from build123d import *

# Parameters (mm, degrees)
F0_R      = 6.35
F1_DEPTH  = 19.05
F3_D      = 5.08
F8_D      = 3.175
F8_DEPTH  = 2.54
F8_TIP    = 0.9538662327
F9_D      = 3.175
F9_DEPTH  = 2.54
F9_TIP    = 0.9538662327
F11_D     = 11.938
F11_DEPTH = 12.7
F11_TIP   = 3.586537035


# Not quite as in the source:
# - the program builds the solid bodies; features that only make, move or delete a surface that nothing else refers to are left out


with BuildPart() as f1:
    # F0 (on Top) → F1 (new body)
    with BuildSketch(Plane.XY):
        Circle(F0_R)
    extrude(amount=F1_DEPTH)

    # F3 (through all)
    with Locations(Plane(origin=(0, 0, 0), x_dir=(1, 0, 0), z_dir=(0, 0, -1))):
        with Locations((0, 0)):
            Hole(F3_D / 2)

    # F8
    with Locations(Plane.XY.offset(19.05)):
        with Locations((0, 4.4337138534)):
            Hole(F8_D / 2, depth=F8_DEPTH)
            with Locations((0, 0, -(F8_DEPTH + F8_TIP / 2))):  # 118° drill point
                Cone(0, F8_D / 2, F8_TIP, mode=Mode.SUBTRACT)

    # F9
    with Locations(Plane.XY.offset(19.05)):
        with Locations((0, -4.445)):
            Hole(F9_D / 2, depth=F9_DEPTH)
            with Locations((0, 0, -(F9_DEPTH + F9_TIP / 2))):  # 118° drill point
                Cone(0, F9_D / 2, F9_TIP, mode=Mode.SUBTRACT)

    # F11
    with Locations(Plane(origin=(0, 0, 0), x_dir=(1, 0, 0), z_dir=(0, 0, -1))):
        with Locations((0, 0)):
            Hole(F11_D / 2, depth=F11_DEPTH)
            with Locations((0, 0, -(F11_DEPTH + F11_TIP / 2))):  # 118° drill point
                Cone(0, F11_D / 2, F11_TIP, mode=Mode.SUBTRACT)


solid = f1.part
The listing builds one solid part. Answer for the finished solid, in the listing's coordinates (mm). A direction names the side the tool comes from. Give positions to 0.01 mm unless a question says otherwise; leave off trailing zeros. Write each loop counter-clockwise with the first axis right and the second up, starting at its lowest first coordinate (ties: lowest second). Pieces come first, ordered by that corner, then holes. Notation, with made-up numbers: (81.25, -30) -> (112.25, -30) arc R28 cw to (112.25, 1) -> close; hole circle Ø10 at (51.5, 43.25). An arc over 180 degrees is marked (long way). Use a Markdown table: item, result.
(1) Find the intervals of material crossed by probe 1 along Y at (x, z) = (0, 17.9); probe 2 along Y at (x, z) = (0, 3.5); probe 3 along Y at (x, z) = (0, 15.9), in increasing order. Write a range as from..to.
Return value:
| item | result |
|---|---|
| probe 1 | -6.35..-6.03, -2.86..-2.54, 2.54..2.85, 6.02..6.35 |
| probe 2 | -6.35..-5.97, 5.97..6.35 |
| probe 3 | -6.35..-5.02, -3.87..-2.54, 2.54..3.86, 5.01..6.35 |
(2) Section A-A, the plane y = 0 is taken. Determine the outline of the cut face in (x, z).
Return value:
| item | result |
|---|---|
| outline | (-6.35, 0) -> (-5.97, 0) -> (-5.97, 12.7) -> (-2.54, 14.76) -> (-2.54, 19.05) -> (-6.35, 19.05) -> close; (2.54, 14.76) -> (5.97, 12.7) -> (5.97, 0) -> (6.35, 0) -> (6.35, 19.05) -> (2.54, 19.05) -> close |
(3) Determine the mould class of faces 4 (the cylindrical face through (0.344, 2.884, 17.762)), 5 (the flat face through (-0.1, -2.7, 19.05)), 6 (the cylindrical face through (-1.38, -6.2, 9.39)) for opening direction X: released by +X, released by -X, zero draft, split by the parting line, or undercut.
Return value:
| item | result |
|---|---|
| face 4 | undercut |
| face 5 | zero draft |
| face 6 | split by the parting line |
(4) Section B-B, the plane z = 4.75 is taken. Determine the outline of the cut face in (x, y), then the cut area to 3 significant figures.
Return value:
| item | result |
|---|---|
| outline | circle Ø12.7 at (0, 0); hole circle Ø11.94 at (0, 0) |
| area | 14.7 mm2 |
(5) For faces 1 (the cylindrical face through (1.294, 5.827, 6.439)), 2 (the cylindrical face through (-0.733, -5.853, 17.762)), 3 (the cylindrical face through (0.33, -2.52, 16.94)), determine the directions among +Z, -Z, +X, -X, +Y, -Y from which every point of the face is accessible in a straight line to the end or side of a thin tool.
Return value:
| item | result |
|---|---|
| face 1 | -Z |
| face 2 | +Z |
| face 3 | +Z, -Z |
(6) Flat-ended cylindrical pins translate along their axes: P1, Ø3, axis at y = 4.5, z = 3.5, coming from the -X side; P2, Ø1, axis at x = -1, z = 4, coming from the -Y side; P3, Ø7, axis at x = 0, y = 0, coming from the -Z side. Find the tip coordinate at first contact, or state that the pin passes through.
Return value:
| item | result |
|---|---|
| P1 | x = -5.6 |
| P2 | y = -6.33 |
| P3 | z = 14.18 |
